```python
from build123d import *

# Parameters (mm, degrees)
SKETCH1_W               = 60
SKETCH1_H               = 60
SKETCH1_W_2             = 54
SKETCH1_H_2             = 54
BOSS_EXTRUDE1_DEPTH     = 250
FILLET1_R               = 3
SKETCH2_R               = 2
SKETCH2_R_2             = 2.25
SKETCH2_R_3             = 12.5
SKETCH2_R_4             = 14
CUT_EXTRUDE1_DEPTH      = 31
CUT_EXTRUDE1_DEPTH_BACK = 31


with BuildPart() as part:
    # Sketch1 → Boss-Extrude1 (new body)
    with BuildSketch(Plane.XY):
        Rectangle(SKETCH1_W, SKETCH1_H)
        Rectangle(SKETCH1_W_2, SKETCH1_H_2, mode=Mode.SUBTRACT)
    extrude(amount=BOSS_EXTRUDE1_DEPTH)

    # Fillet1
    fillet1_edges = [part.edges().sort_by_distance(p)[0] for p in [
        (27, -27, 125),
        (27, 27, 125),
        (-27, 27, 125),
        (-27, -27, 125),
        (30, -30, 125),
        (-30, -30, 125),
        (-30, 30, 125),
        (30, 30, 125),
    ]]
    fillet(fillet1_edges, radius=FILLET1_R)

    # Sketch2 → Cut-Extrude1 (cut, two sides)
    with BuildSketch(Plane(origin=(0, 0, 0), x_dir=(1, 0, 0), z_dir=(0, 1, 0))) as cut_extrude1_sk:
        with Locations((0, -142)):
            Circle(SKETCH2_R)
        with Locations((-14.722431864, -133.5)):
            Circle(SKETCH2_R)
        with Locations((-14.722431864, -116.5)):
            Circle(SKETCH2_R)
        with Locations((0, -108)):
            Circle(SKETCH2_R)
        with Locations((14.722431864, -116.5)):
            Circle(SKETCH2_R)
        with Locations((14.722431864, -133.5)):
            Circle(SKETCH2_R)
        with Locations((-13.435028843, -216.564971157)):
            Circle(SKETCH2_R_2)
        with Locations((13.435028843, -216.564971157)):
            Circle(SKETCH2_R_2)
        with Locations((13.435028843, -243.435028843)):
            Circle(SKETCH2_R_2)
        with Locations((-13.435028843, -243.435028843)):
            Circle(SKETCH2_R_2)
        with Locations((-13.435028843, -6.564971157)):
            Circle(SKETCH2_R_2)
        with Locations((13.435028843, -6.564971157)):
            Circle(SKETCH2_R_2)
        with Locations((13.435028843, -33.435028843)):
            Circle(SKETCH2_R_2)
        with Locations((-13.435028843, -33.435028843)):
            Circle(SKETCH2_R_2)
        with Locations((0, -125)):
            Circle(SKETCH2_R_3)
        with Locations((0, -230)):
            Circle(SKETCH2_R_4)
        with Locations((0, -20)):
            Circle(SKETCH2_R_4)
    extrude(amount=CUT_EXTRUDE1_DEPTH, mode=Mode.SUBTRACT)
    extrude(cut_extrude1_sk.sketch, amount=-CUT_EXTRUDE1_DEPTH_BACK, mode=Mode.SUBTRACT)


solid = part.part
```
Model file for the job. Use its own axes, mm. Coordinates: 2 decimals unless noted, no trailing zeros. Order: outer loops, then holes, each group sorted by start corner. A loop starts at its lowest first (then second) coordinate and runs counter-clockwise, first axis right, second up. Notation, with made-up numbers: (7.5, 60) - (19.5, 60) arc R25 cw to (19.5, 99) - close; hole circle Ø2 at (25.5, -31). An arc over 180 degrees is marked (long way). Return JSON: item names as keys, results as strings. Group by question number.
1) Mould opens along Z. For faces 1 (the cylindrical face through (1.075, 28.479, 106.314)), 2 (the cylindrical face through (12.947, -28.479, 245.632)), 3 (the flat face through (0, 29, 0)), 4 (the flat face through (-16, 27, 123)) say: released by +Z, released by -Z, zero draft, split by the parting line, or undercut.
2) Saw through at A-A, the plane x = -20. Write the cut outline in (y, z), plus the area to 3 significant figures.
3) Probe line 1 (Z direction, x = 0, y = 28.5); line 2 (X direction, y = -2, z = 177). List the from-to ranges inside material, lowest first. Write a range as from..to.
4) Saw through at B-B, the plane z = 125. Write the cut outline in (x, y).
5) Saw through at D-D, the plane z = 159.5. Write the cut outline in (x, y).
Values found:
{
 "1": {"face 1": "undercut", "face 2": "undercut", "face 3": "released by -Z", "face 4": "zero draft"},
 "2": {"outline": "(-30, 0) - (-27, 0) - (-27, 250) - (-30, 250) - close; (27, 0) - (30, 0) - (30, 250) - (27, 250) - close", "area": "1,500 mm²"},
 "3": {"line 1": "z = 0..6, 34..106, 110..112.5, 137.5..140, 144..216, 244..250", "line 2": "x = -30..-27, 27..30"},
 "4": {"outline": "(-30, -27) arc R3 ccw to (-27, -30) - (-12.5, -30) - (-12.5, -27) - (-24, -27) arc R3 cw to (-27, -24) - (-27, 24) arc R3 cw to (-24, 27) - (-12.5, 27) - (-12.5, 30) - (-27, 30) arc R3 ccw to (-30, 27) - close; (12.5, -30) - (27, -30) arc R3 ccw to (30, -27) - (30, 27) arc R3 ccw to (27, 30) - (12.5, 30) - (12.5, 27) - (24, 27) arc R3 cw to (27, 24) - (27, -24) arc R3 cw to (24, -27) - (12.5, -27) - close"},
 "5": {"outline": "(-30, -27) arc R3 ccw to (-27, -30) - (27, -30) arc R3 ccw to (30, -27) - (30, 27) arc R3 ccw to (27, 30) - (-27, 30) arc R3 ccw to (-30, 27) - close; hole (-27, -24) arc R3 ccw to (-24, -27) - (24, -27) arc R3 ccw to (27, -24) - (27, 24) arc R3 ccw to (24, 27) - (-24, 27) arc R3 ccw to (-27, 24) - close"}
}
